Geometry: final body of the model. Coordinates: model frame, mm. Coordinates: 2 decimals unless noted, no trailing zeros. Order: outer loops, then holes, each group sorted by start corner. A loop starts at its lowest first (then second) coordinate and runs counter-clockwise, first axis right, second up. Notation, with made-up numbers: M 21,21 L 51,21 A16 ccw 51,47 Z; hole C 23.25,65.25 d1. An arc over 180 degrees is marked long. Write item = value, one per line.
from build123d import *

# Parameters (mm, degrees)
SKETCH_1_R      = 1.6
EXTRUDE_1_DEPTH = 1.5
FILLET_1_R      = 2


with BuildPart() as part:
    # ｽｹｯﾁ1 → ﾎﾞｽ - 押し出し1 (new body)
    with BuildSketch(Plane.XY):
        Polygon((-5, 60), (-22.5, 20), (-22.5, 10), (-5, -10), (5, -10), (22.5, 10), (22.5, 20), (5, 60), align=None)
        Circle(SKETCH_1_R, mode=Mode.SUBTRACT)
        with Locations((0, 50)):
            Circle(SKETCH_1_R, mode=Mode.SUBTRACT)
        with Locations((-17.5, 15)):
            Circle(SKETCH_1_R, mode=Mode.SUBTRACT)
        with Locations((17.5, 15)):
            Circle(SKETCH_1_R, mode=Mode.SUBTRACT)
    extrude(amount=EXTRUDE_1_DEPTH)

    # ﾌｨﾚｯﾄ1
    fillet_1_edges = [part.edges().sort_by_distance(p)[0] for p in [
        (22.5, 20, 0.75),
        (22.5, 10, 0.75),
        (5, -10, 0.75),
        (-5, -10, 0.75),
        (-22.5, 10, 0.75),
        (-22.5, 20, 0.75),
        (-5, 60, 0.75),
        (5, 60, 0.75),
    ]]
    fillet(fillet_1_edges, radius=FILLET_1_R)


solid = part.part
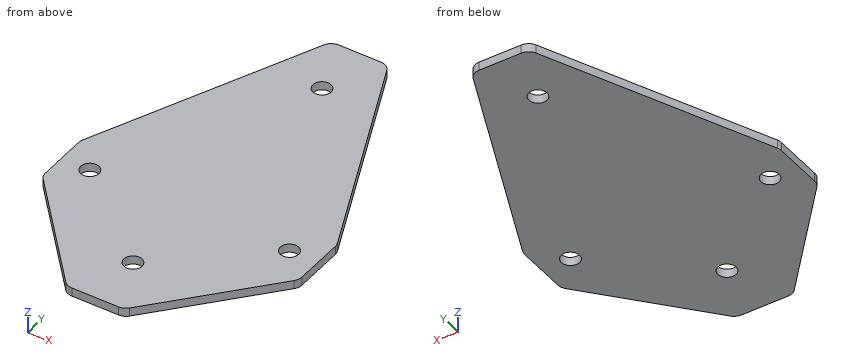
1) Section D-D, the plane y = 50. Return loops of the section in (x, z) (3 decimals), and give its area (3 significant figures).
Numbers:
outline = M -9.375,0 L -1.6,0 L -1.6,1.5 L -9.375,1.5 Z; M 1.6,0 L 9.375,0 L 9.375,1.5 L 1.6,1.5 Z
area = 23.3 mm²
2) Section B-B, the plane z = 1.15. Return loops of the section in (x, y), and give its area (3 significant figures).
Numbers:
outline = M -22.5,10.75 A2 ccw -22.01,9.43 L -5.6,-9.32 A2 ccw -4.09,-10 L 4.09,-10 A2 ccw 5.6,-9.32 L 22.01,9.43 A2 ccw 22.5,10.75 L 22.5,19.58 A2 ccw 22.33,20.38 L 5.52,58.8 A2 ccw 3.69,60 L -3.69,60 A2 ccw -5.52,58.8 L -22.33,20.38 A2 ccw -22.5,19.58 Z; hole C -17.5,15 d3.2; hole C 0,0 d3.2; hole C 0,50 d3.2; hole C 17.5,15 d3.2
area = 2,070 mm²
3) Line query: L1, parallel to Y at x = 0, z = 0.9; L2, parallel to X at y = 16, z = 1.05; L3, parallel to Y at x = -0.5, z = 1.1. Output: solid intervals per line, ascending.
Numbers:
L1 = -10 to -1.6, 1.6 to 48.4, 51.6 to 60
L2 = -22.5 to -18.75, -16.25 to 16.25, 18.75 to 22.5
L3 = -10 to -1.52, 1.52 to 48.48, 51.52 to 60
4) Pin query (flat end, axial travel): pin 1 (3 mm diameter, centred on x = 0, y = 50, fed in from +Z). Return the tip coordinate at first contact, or that it passes through.
Numbers:
pin_1 = through
5) Section C-C, the plane x = -18. Return loops of the section in (y, z), and give its area (3 significant figures).
Numbers:
outline = M 4.86,0 L 13.48,0 L 13.48,1.5 L 4.86,1.5 Z; M 16.52,0 L 30.29,0 L 30.29,1.5 L 16.52,1.5 Z
area = 33.6 mm²
6) Section A-A, the plane y = 15. Return loops of the section in (x, z).
Numbers:
outline = M -22.5,0 L -19.1,0 L -19.1,1.5 L -22.5,1.5 Z; M -15.9,0 L 15.9,0 L 15.9,1.5 L -15.9,1.5 Z; M 19.1,0 L 22.5,0 L 22.5,1.5 L 19.1,1.5 Z
